Work out the finished part from the listing and answer in its coordinate system (mm). Face numbers are marked on the shaded views. A direction names the side the tool comes from. Round coordinates to 2 decimals unless told otherwise and drop trailing zeros. Loops run counter-clockwise (first coordinate to the right, second up) from the corner with the lowest first, then second, coordinate; pieces in that order, holes last.
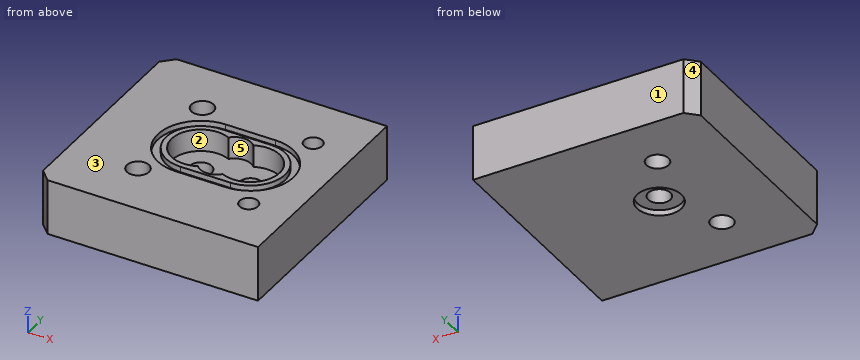
from build123d import *

# Parameters (mm, degrees)
F0_W      = 41
F0_H      = 40
F0_R      = 2
F0_R_2    = 1.65
F1_DEPTH  = 10
F2_DEPTH  = 1
F3_DEPTH  = 8
F4_DEPTH  = 4
F5_R      = 4
F5_R_2    = 2
F6_DEPTH  = 1
F7_DEPTH  = 8
F8_DEPTH  = 2
F9_SIZE   = 2
F10_DEPTH = 3


# Not quite as in the source:
# - a feature names something its author has since deleted; it is built from what else it names


with BuildPart() as f1:
    # F0 (on Top) → F1 (new body)
    with BuildSketch(Plane.XY):
        with Locations((20.5, -20)):
            Rectangle(F0_W, F0_H)
        with Locations((10.5, -30)):
            Circle(F0_R, mode=Mode.SUBTRACT)
        with Locations((30.5, -30)):
            Circle(F0_R_2, mode=Mode.SUBTRACT)
        with Locations((10.5, -10)):
            Circle(F0_R, mode=Mode.SUBTRACT)
        with BuildLine():
            Line((25, -27.75), (16, -27.75))
            ThreePointArc((16, -27.75), (8.25, -20), (16, -12.25))
            Line((16, -12.25), (25, -12.25))
            ThreePointArc((25, -12.25), (32.75, -20), (25, -27.75))
        make_face(mode=Mode.SUBTRACT)
        with Locations((30.5, -10)):
            Circle(F0_R_2, mode=Mode.SUBTRACT)
        with BuildLine():
            ThreePointArc((16, -12.25), (8.25, -20), (16, -27.75))
            Line((16, -27.75), (25, -27.75))
            ThreePointArc((25, -27.75), (32.75, -20), (25, -12.25))
            Line((25, -12.25), (16, -12.25))
        make_face()
        with BuildLine():
            ThreePointArc((16, -26.25), (9.75, -20), (16, -13.75))
            Line((16, -13.75), (25, -13.75))
            ThreePointArc((25, -13.75), (31.25, -20), (25, -26.25))
            Line((25, -26.25), (16, -26.25))
        make_face(mode=Mode.SUBTRACT)
        with BuildLine():
            Line((25, -13.75), (16, -13.75))
            ThreePointArc((16, -13.75), (9.75, -20), (16, -26.25))
            Line((16, -26.25), (25, -26.25))
            ThreePointArc((25, -26.25), (31.25, -20), (25, -13.75))
        make_face()
        with BuildLine():
            ThreePointArc((22.7443308628, -15.25927677), (30.25, -20), (22.7443308628, -24.74072323))
            ThreePointArc((22.7443308628, -24.74072323), (20.5, -25.75), (18.2556691372, -24.74072323))
            ThreePointArc((18.2556691372, -24.74072323), (10.75, -20), (18.2556691372, -15.25927677))
            ThreePointArc((18.2556691372, -15.25927677), (20.5, -14.25), (22.7443308628, -15.25927677))
        make_face(mode=Mode.SUBTRACT)
        with BuildLine():
            ThreePointArc((18.2556691372, -24.74072323), (20.5, -25.75), (22.7443308628, -24.74072323))
            ThreePointArc((22.7443308628, -24.74072323), (30.25, -20), (22.7443308628, -15.25927677))
            ThreePointArc((22.7443308628, -15.25927677), (20.5, -14.25), (18.2556691372, -15.25927677))
            ThreePointArc((18.2556691372, -15.25927677), (10.75, -20), (18.2556691372, -24.74072323))
        make_face()
        with Locations((16, -20)):
            Circle(F0_R, mode=Mode.SUBTRACT)
        with Locations((25, -20)):
            Circle(F0_R, mode=Mode.SUBTRACT)
        with Locations((25, -20)):
            Circle(F0_R)
        with Locations((30.5, -10)):
            Circle(F0_R_2)
        with Locations((30.5, -30)):
            Circle(F0_R_2)
    extrude(amount=-F1_DEPTH)

    # F0 (on Top) → F2 (cut)
    with BuildSketch(Plane.XY):
        with BuildLine():
            ThreePointArc((16, -12.25), (8.25, -20), (16, -27.75))
            Line((16, -27.75), (25, -27.75))
            ThreePointArc((25, -27.75), (32.75, -20), (25, -12.25))
            Line((25, -12.25), (16, -12.25))
        make_face()
        with BuildLine():
            ThreePointArc((16, -26.25), (9.75, -20), (16, -13.75))
            Line((16, -13.75), (25, -13.75))
            ThreePointArc((25, -13.75), (31.25, -20), (25, -26.25))
            Line((25, -26.25), (16, -26.25))
        make_face(mode=Mode.SUBTRACT)
    extrude(amount=-F2_DEPTH, mode=Mode.SUBTRACT)

    # F0 (on Top) → F3 (cut)
    with BuildSketch(Plane.XY):
        with Locations((25, -20)):
            Circle(F0_R)
    extrude(amount=-F3_DEPTH, mode=Mode.SUBTRACT)

    # F0 (on Top) → F4 (cut)
    with BuildSketch(Plane.XY):
        with BuildLine():
            ThreePointArc((18.2556691372, -24.74072323), (20.5, -25.75), (22.7443308628, -24.74072323))
            ThreePointArc((22.7443308628, -24.74072323), (30.25, -20), (22.7443308628, -15.25927677))
            ThreePointArc((22.7443308628, -15.25927677), (20.5, -14.25), (18.2556691372, -15.25927677))
            ThreePointArc((18.2556691372, -15.25927677), (10.75, -20), (18.2556691372, -24.74072323))
        make_face()
        with Locations((16, -20)):
            Circle(F0_R, mode=Mode.SUBTRACT)
        with Locations((25, -20)):
            Circle(F0_R, mode=Mode.SUBTRACT)
    extrude(amount=-F4_DEPTH, mode=Mode.SUBTRACT)

    # F5 (on face) → F6 (cut)
    with BuildSketch(Plane(origin=(0, 0, -10), x_dir=(1, 0, 0), z_dir=(0, 0, -1))):
        with Locations((16, 20)):
            Circle(F5_R)
        with Locations((16, 20)):
            Circle(F5_R_2, mode=Mode.SUBTRACT)
    extrude(amount=-F6_DEPTH, mode=Mode.SUBTRACT)

    # F0 (on Top) → F7 (cut)
    with BuildSketch(Plane.XY):
        with Locations((30.5, -30)):
            Circle(F0_R_2)
        with Locations((30.5, -10)):
            Circle(F0_R_2)
    extrude(amount=-F7_DEPTH, mode=Mode.SUBTRACT)

    # F8 (add): a face of the model
    f8_faces = [f1.faces().sort_by_distance(p)[0] for p in [
        (0, -20, -5),
    ]]
    extrude(f8_faces, amount=F8_DEPTH)

    # F9
    f9_edges = [f1.edges().sort_by_distance(p)[0] for p in [
        (-2, -40, -5),
        (-2, 0, -5),
    ]]
    chamfer(f9_edges, length=F9_SIZE)

    # F10 (cut): a face of the model
    f10_faces = [f1.faces().sort_by_distance(p)[0] for p in [
        (41, -20, -5),
    ]]
    extrude(f10_faces, amount=-F10_DEPTH, mode=Mode.SUBTRACT)


solid = f1.part
Item 1: Section C-C, the plane z = -6.5 is taken. Give the vertices of the cut face in (x, y).
Item 2: Section D-D, the plane y = -20 is taken. Give the vertices of the cut face in (x, z).
Item 3: Each of these flat-tipped pins is pushed along its axis until it touches: P1, Ø3.5, axis at x = 10.5, y = -30, coming from the -Z side; P2, Ø4.5, axis at x = 24.5, y = -19.5, coming from the +Z side; P3, Ø7, axis at x = 16, y = -20, coming from the -Z side; P4, Ø1.6, axis at x = 30.5, y = -29.5, coming from the +Z side. Where does it stop, or does it pass through?
Item 4: Section B-B, the plane z = -2.75 is taken. Give the vertices of the cut face in (x, y).
Item 5: Straight lines are drawn through the part: line 1 (Y direction, x = 10.5, z = -9.25); line 2 (X direction, y = -20, z = -0.75); line 3 (Y direction, x = 25, z = -5). For each, find the intervals that lie inside material, in ascending order.
Item 6: For the marked faces 1 and 2, determine the directions among +Z, -Z, +X, -X, +Y, -Y from which every point of the face is accessible in a straight line to the end or side of a thin tool.
Item 7: Determine the mould class of the marked faces 3, 4 and 5 for opening direction X: pulls with the +X half, pulls with the -X half, needs draft (parallel to the pull), parting line crosses it, or undercut.
Item 8: Section A-A, the plane y = -30 is taken. Give the vertices of the cut face in (x, z), plus the area to 3 significant figures.
Answer below:
1. outline: (-2, -38) - (0, -40) - (38, -40) - (38, 0) - (0, 0) - (-2, -2) - close; hole circle Ø4 at (10.5, -30); hole circle Ø4 at (10.5, -10); hole circle Ø4 at (16, -20); hole circle Ø4 at (25, -20); hole circle Ø3.3 at (30.5, -30); hole circle Ø3.3 at (30.5, -10)
2. outline: (-2, -10) - (12, -10) - (12, -9) - (14, -9) - (14, -4) - (10.75, -4) - (10.75, 0) - (9.75, 0) - (9.75, -1) - (8.25, -1) - (8.25, 0) - (-2, 0) - close; (18, -9) - (20, -9) - (20, -10) - (38, -10) - (38, 0) - (32.75, 0) - (32.75, -1) - (31.25, -1) - (31.25, 0) - (30.25, 0) - (30.25, -4) - (27, -4) - (27, -8) - (23, -8) - (23, -4) - (18, -4) - close
3. P1: passes through
3. P2: stops at z = -4
3. P3: stops at z = -9
3. P4: stops at z = -8
4. outline: (-2, -38) - (0, -40) - (38, -40) - (38, 0) - (0, 0) - (-2, -2) - close; hole circle Ø4 at (10.5, -30); hole circle Ø4 at (10.5, -10); hole (18.26, -24.74) arc R3 ccw to (22.74, -24.74) arc R5.25 ccw (long way) to (22.74, -15.26) arc R3 ccw to (18.26, -15.26) arc R5.25 ccw (long way) to start; hole circle Ø3.3 at (30.5, -30); hole circle Ø3.3 at (30.5, -10)
5. line 1: y = -40 to -32, -28 to -12, -8 to 0
5. line 2: x = -2 to 8.25, 9.75 to 10.75, 30.25 to 31.25, 32.75 to 38
5. line 3: y = -40 to -22, -18 to 0
6. face 1: +Z, -Z, +X, -X, +Y
6. face 2: +Z
7. face 3: needs draft
7. face 4: pulls with the -X half
7. face 5: undercut
8. outline: (-2, -10) - (8.5, -10) - (8.5, 0) - (-2, 0) - close; (12.5, -10) - (38, -10) - (38, 0) - (32.15, 0) - (32.15, -8) - (28.85, -8) - (28.85, 0) - (12.5, 0) - close
8. area: 334 mm2
